Read the model definition and answer for the solid it produces. Units are mm, in the model's axes. A direction names the side the tool comes from. Round coordinates to 2 decimals unless told otherwise and drop trailing zeros. Order: outer loops, then holes, each group sorted by start corner. A loop starts at its lowest first (then second) coordinate and runs counter-clockwise, first axis right, second up. Notation, with made-up numbers: (-8.5, 4) -> (26.5, 4) arc R24 cw to (26.5, 20) -> close; hole circle Ø4 at (-33.75, 74). An arc over 180 degrees is marked (long way). One line per item, written item: value. Start each with the question number.
1. For faces 1 (the face through (-4.609, 22.807, -8.134)), 2 (the face through (8.5, 26.67, -4.9)), 3 (the face through (-4, 19.05, -5)), determine the directions among +Z, -Z, +X, -X, +Y, -Y from which every point of the face is accessible in a straight line to the end or side of a thin tool.
2. Flat-ended cylindrical pins translate along their axes: pin 1 Ø1.5 at (x, z) = (-4.5, -8.5) entering from -Y; pin 2 Ø3.5 at (x, z) = (-7, -4) entering from +Y; pin 3 Ø4 at (x, y) = (6, 32.5) entering from -Z; pin 4 Ø4 at (y, z) = (22, 1) entering from -X. Find the tip coordinate at first contact, or state that the pin passes through.
3. Section C-C (y = 6.5) is taken. Give the vertices of the cut face in (x, z).
4. Section D-D (z = 6.5) is taken. Give the vertices of the cut face in (x, y) (3 decimals), then the cut area to 3 significant figures.
5. Section A-A (z = 0) is taken. Give the vertices of the cut face in (x, y) (3 decimals), then the cut area to 3 significant figures.
6. Section B-B (x = 0.5) is taken. Give the vertices of the cut face in (y, z) (3 decimals).
7. Consider line 1 (X direction, y = 22.5, z = -0.5); line 2 (Y direction, x = 7.25, z = -5.25) (3 decimals); line 3 (Y direction, x = -2.75, z = -7.25). Determine where each line is inside the solid, lowest interval first.
from build123d import *

# Parameters (mm, degrees)
CUT_EXTRUDE1_DEPTH = 7.62


with BuildPart() as part:
    # Sketch1 → Revolve1 (revolve)
    with BuildSketch(Plane.XY):
        Polygon((0, 0), (5.55625, 0), (5.55625, 19.05), (10.795, 19.05), (10.795, 26.67), (9.525, 26.67), (9.525, 36.195), (7.874, 36.195), (7.874, 46.99), (0, 46.99), align=None)
    revolve(axis=Axis((0, 46.99, 0), (0, -1, 0)))

    # Sketch2 → Cut-Extrude1 (cut)
    with BuildSketch(Plane.XZ.offset(-19.05)):
        with BuildLine():
            Line((-9.348744234, 5.3975), (0, 10.795))
            ThreePointArc((0, 10.795), (-5.3975, 9.348744234), (-9.348744234, 5.3975))
        make_face()
        with BuildLine():
            ThreePointArc((9.348744234, 5.3975), (5.3975, 9.348744234), (0, 10.795))
            Line((0, 10.795), (9.348744234, 5.3975))
        make_face()
        with BuildLine():
            ThreePointArc((10.795, 0), (10.427169295, 2.793951592), (9.348744234, 5.3975))
            Line((9.348744234, 5.3975), (9.348744234, -5.3975))
            ThreePointArc((9.348744234, -5.3975), (10.427169295, -2.793951592), (10.795, 0))
        make_face()
        with BuildLine():
            ThreePointArc((0, -10.795), (5.3975, -9.348744234), (9.348744234, -5.3975))
            Line((9.348744234, -5.3975), (0, -10.795))
        make_face()
        with BuildLine():
            Line((0, -10.795), (-9.348744234, -5.3975))
            ThreePointArc((-9.348744234, -5.3975), (-5.3975, -9.348744234), (0, -10.795))
        make_face()
        with BuildLine():
            Line((-9.348744234, -5.3975), (-9.348744234, 5.3975))
            ThreePointArc((-9.348744234, 5.3975), (-10.795, 0), (-9.348744234, -5.3975))
        make_face()
    extrude(amount=-CUT_EXTRUDE1_DEPTH, mode=Mode.SUBTRACT)


solid = part.part
Answer:
1. face 1: -Z, -X, -Y
1. face 2: -Z, +X, +Y
1. face 3: -Y
2. pin 1: y = 19.05
2. pin 2: y = 46.99
2. pin 3: z = -8.64
2. pin 4: x = -9.35
3. outline: circle Ø11.11 at (0, 0)
4. outline: (-7.439, 19.05) -> (7.439, 19.05) -> (7.439, 26.67) -> (6.962, 26.67) -> (6.962, 36.195) -> (4.444, 36.195) -> (4.444, 46.99) -> (-4.444, 46.99) -> (-4.444, 36.195) -> (-6.962, 36.195) -> (-6.962, 26.67) -> (-7.439, 26.67) -> close
4. area: 342 mm^2
5. outline: (-9.525, 26.67) -> (-9.349, 26.67) -> (-9.349, 19.05) -> (-5.556, 19.05) -> (-5.556, 0) -> (5.556, 0) -> (5.556, 19.05) -> (9.349, 19.05) -> (9.349, 26.67) -> (9.525, 26.67) -> (9.525, 36.195) -> (7.874, 36.195) -> (7.874, 46.99) -> (-7.874, 46.99) -> (-7.874, 36.195) -> (-9.525, 36.195) -> close
5. area: 706 mm^2
6. outline: (0, -5.534) -> (19.05, -5.534) -> (19.05, -10.506) -> (26.67, -10.506) -> (26.67, -9.512) -> (36.195, -9.512) -> (36.195, -7.858) -> (46.99, -7.858) -> (46.99, 7.858) -> (36.195, 7.858) -> (36.195, 9.512) -> (26.67, 9.512) -> (26.67, 10.506) -> (19.05, 10.506) -> (19.05, 5.534) -> (0, 5.534) -> close
7. line 1: -9.35 to 9.35
7. line 2: 19.05 to 36.195
7. line 3: 19.05 to 46.99
